CAD build for the part. Positions are in the model's coordinates, mm. A direction names the side the tool comes from. Coordinates: 2 decimals unless noted, no trailing zeros. Write each loop counter-clockwise with the first axis right and the second up, starting at its lowest first coordinate (ties: lowest second). Pieces come first, ordered by that corner, then holes. Notation, with made-up numbers: (9.25, 32) - (56.25, 32) arc R15 cw to (56.25, 53) - close; hole circle Ø10 at (84.5, 38.25). An arc over 180 degrees is marked (long way). Answer in a Markdown table with one row per item. Add a question column.
Q1. Two-plate mould, pull along X, no slides. Class faces 1 (the flat face through (-14.33, 3, 2)), 2 (the flat face through (3.6, 3.556, 1.6)), 3 (the flat face through (-4, 1.016, 2)), 4 (the flat face through (-3.4, 0.4, 0)): +X half, -X half, draft (parallel to the pull), parting line (faces both ways), or undercut.
Q2. Drill centre lines: line 1 along X through (y, z) = (2.5, 1.05); line 2 along X through (y, z) = (4.25, 2.45); line 3 along Y through (x, z) = (0, 1.7). Where is each one in solid material? Low to high. Write a range as from..to.
Q3. Band-saw the part on D-D (x = -9). List the corners of the cut face in (y, z) (3 decimals), and give its area (3 significant figures).
Q4. 3-axis set-ups, long thin cutter, end or side, ignore diameter. For faces 5 (the flat face through (3.069, 2, 2)), 6 (the flat face through (-12.171, 4, 2)), 7 (the flat face through (-13, 7.112, 2)): which of +Z, -Z, +X, -X, +Y, -Y reach the whole face in a straight line?
Q5. Band-saw the part on A-A (y = 6). List the corners of the cut face in (x, z) (3 decimals).
Q6. Pin check, flat tips, straight feed: pin 1 (0.7 mm diameter, centred on x = -1, z = 1.5, fed in from +Y); pin 2 (2 mm diameter, centred on x = -6, y = 3, fed in from -Z). Stop position of each tip, or through.
Q7. Band-saw the part on C-C (y = 4). List the corners of the cut face in (x, z) (3 decimals), and give its area (3 significant figures).
Q8. Band-saw the part on B-B (z = 2.1). List the corners of the cut face in (x, y).
```python
from build123d import *

# Parameters (mm, degrees)
F1_DEPTH = 3.175
F2_R     = 0.508
F3_R     = 0.381


with BuildPart() as f1:
    # F0 (on Top) → F1 (new body)
    with BuildSketch(Plane.XY):
        Polygon((-14.330484, 1.016), (-14.330484, 0), (6.243516, 0), (6.243516, 1.016), (6.243516, 7.112), (3.068516, 7.112), (3.068516, 5.334), (4.084516, 5.334), (4.084516, 3.556), (3.068516, 3.556), (3.068516, 1.016), (-11.155484, 1.016), (-11.155484, 3.556), (-12.171484, 3.556), (-12.171484, 5.334), (-11.155484, 5.334), (-11.155484, 7.112), (-14.330484, 7.112), align=None)
    extrude(amount=F1_DEPTH)

    # F2
    f2_edges = [f1.edges().sort_by_distance(p)[0] for p in [
        (-11.155484, 2.286, 3.175),
        (-11.155484, 2.286, 0),
        (3.068516, 2.286, 3.175),
        (6.243516, 3.556, 3.175),
        (6.243516, 3.556, 0),
        (-14.330484, 3.556, 3.175),
        (-12.742984, 7.112, 3.175),
        (6.243516, 7.112, 1.5875),
        (4.656016, 7.112, 3.175),
        (4.656016, 7.112, 0),
        (3.068516, 7.112, 1.5875),
        (-11.155484, 7.112, 1.5875),
        (-12.742984, 7.112, 0),
        (-14.330484, 7.112, 1.5875),
        (-11.155484, 6.223, 3.175),
        (-11.155484, 6.223, 0),
        (3.068516, 6.223, 3.175),
        (3.068516, 6.223, 0),
        (3.068516, 2.286, 0),
        (-14.330484, 3.556, 0),
    ]]
    fillet(f2_edges, radius=F2_R)

    # F3
    f3_edges = [f1.edges().sort_by_distance(p)[0] for p in [
        (-4.043484, 1.016, 0),
        (-4.043484, 1.016, 3.175),
    ]]
    fillet(f3_edges, radius=F3_R)


solid = f1.part
```
Checked values:
| question | item | result |
|---|---|---|
| 1 | face 1 | -X half |
| 1 | face 2 | undercut |
| 1 | face 3 | undercut |
| 1 | face 4 | draft |
| 2 | line 1 | x = -14.33..-11.16, 3.07..6.24 |
| 2 | line 2 | x = -14.33..-12.17, 4.08..6.24 |
| 2 | line 3 | y = 0..1.02 |
| 3 | outline | (0, 0) - (0.635, 0) arc R0.381 ccw to (1.016, 0.381) - (1.016, 2.794) arc R0.381 ccw to (0.635, 3.175) - (0, 3.175) - close |
| 3 | area | 3.16 mm² |
| 4 | face 5 | +Z, -Z, +Y |
| 4 | face 6 | +Z, -Z |
| 4 | face 7 | +Z, -Z, +X, -X, +Y |
| 5 | outline | (-14.33, 0.508) arc R0.508 ccw to (-13.822, 0) - (-11.663, 0) arc R0.508 ccw to (-11.155, 0.508) - (-11.155, 2.667) arc R0.508 ccw to (-11.663, 3.175) - (-13.822, 3.175) arc R0.508 ccw to (-14.33, 2.667) - close; (3.069, 0.508) arc R0.508 ccw to (3.577, 0) - (5.736, 0) arc R0.508 ccw to (6.244, 0.508) - (6.244, 2.667) arc R0.508 ccw to (5.736, 3.175) - (3.577, 3.175) arc R0.508 ccw to (3.069, 2.667) - close |
| 6 | pin 1 | stops at y = 1.02 |
| 6 | pin 2 | passes through |
| 7 | outline | (-14.33, 0.508) arc R0.508 ccw to (-13.822, 0) - (-12.171, 0) - (-12.171, 3.175) - (-13.822, 3.175) arc R0.508 ccw to (-14.33, 2.667) - close; (4.085, 0) - (5.736, 0) arc R0.508 ccw to (6.244, 0.508) - (6.244, 2.667) arc R0.508 ccw to (5.736, 3.175) - (4.085, 3.175) - close |
| 7 | area | 13.5 mm² |
| 8 | outline | (-14.33, 0) - (6.24, 0) - (6.24, 6.6) arc R0.51 ccw to (5.74, 7.11) - (3.58, 7.11) arc R0.51 ccw to (3.07, 6.6) - (3.07, 5.33) - (4.08, 5.33) - (4.08, 3.56) - (3.07, 3.56) - (3.07, 1.02) - (-11.16, 1.02) - (-11.16, 3.56) - (-12.17, 3.56) - (-12.17, 5.33) - (-11.16, 5.33) - (-11.16, 6.6) arc R0.51 ccw to (-11.66, 7.11) - (-13.82, 7.11) arc R0.51 ccw to (-14.33, 6.6) - close |
